Can you work these out from the drawing? Everything is in mm from the part's minimum corner. Coordinates: 2 decimals unless noted, no trailing zeros. Loops run counter-clockwise (first coordinate to the right, second up) from the corner with the lowest first, then second, coordinate; pieces in that order, holes last. Notation, with made-up numbers: M -18.5,33 L -10.5,33 A22 cw -10.5,62 Z; hole C 23.5,28.25 d6. An arc over 180 degrees is marked long. Use CSV: the item, a comma, the result in double quotes. Start each with the question number.
Q1. If we mould it in two halves opening along Z, with no side actions, what happens to the marked faces 1, 2 and 3? For each: +Z half, -Z half, draft (parallel to the pull), parting line (faces both ways), or undercut.
Q2. If we section it at A-A (x = 25): Please give me the cut outline in (y, z).
Q3. If we section it at B-B (y = 21): Please give me the cut outline in (x, z), and give its area (3 significant figures).
Q4. Please list where these lines run through material, in increasing order: probe 1 along X at (y, z) = (6, 6); probe 2 along Z at (x, y) = (22.5, 6.5); probe 3 along Y at (x, z) = (7, 4). Write a range as [from, to].
Q5. If we section it at C-C (z = 26): Please give me the cut outline in (x, y) (1 decimal), and give its area (3 significant figures).
Q6. For pin 1 Ø4 at (x, z) = (37.37, 5.33) entering from +Y; pin 2 Ø1.9 at (x, z) = (7.5, 17.7) entering from +Y; pin 3 Ø2.5 at (x, z) = (12.63, 5.33) entering from +Y; pin 4 Ø3.5 at (x, y) = (7.5, 6) entering from -Z, each with a flat end and sliding along its axis, tell me the tip position at first contact or that it passes through.
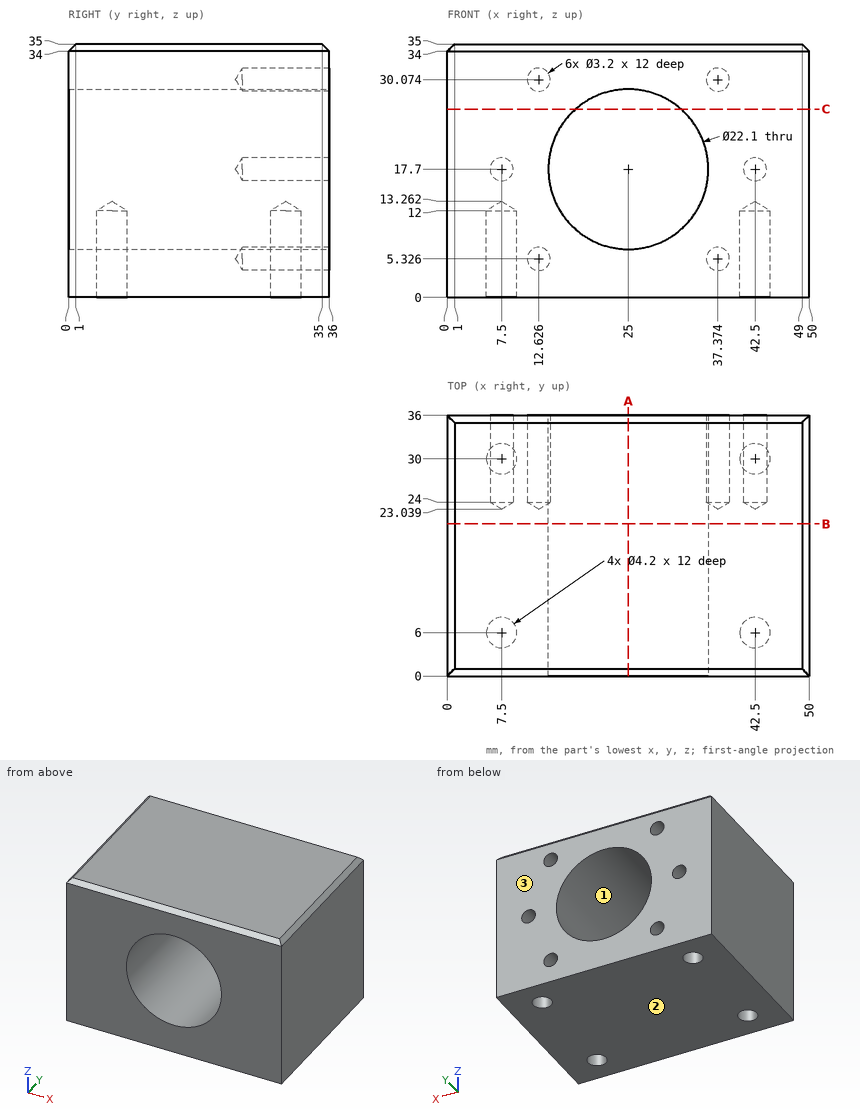
Results below:
1,face 1,"undercut"
1,face 2,"-Z half"
1,face 3,"draft"
2,outline,"M 0,0 L 36,0 L 36,6.65 L 0,6.65 Z; M 0,28.75 L 36,28.75 L 36,34 L 35,35 L 1,35 L 0,34 Z"
3,outline,"M 0,0 L 50,0 L 50,34 L 49,35 L 1,35 L 0,34 Z; hole C 25,17.7 d22.1"
3,area,"1,370 mm^2"
4,probe 1,"[0, 5.4], [9.6, 40.4], [44.6, 50]"
4,probe 2,"[0, 6.94], [28.46, 35]"
4,probe 3,"[0, 3.96], [8.04, 27.96], [32.04, 36]"
5,outline,"M 0,0 L 17.7,0 L 17.7,36 L 0,36 Z; M 32.3,0 L 50,0 L 50,36 L 32.3,36 Z"
5,area,"1,270 mm^2"
6,pin 1,"y = 36"
6,pin 2,"y = 23.61"
6,pin 3,"y = 23.79"
6,pin 4,"z = 12.21"
